Could you check a few things on this model? Use its own coordinates, in mm. A direction names the side the tool comes from. Round coordinates to 2 decimals unless told otherwise and drop trailing zeros. Write each loop counter-clockwise with the first axis right and the second up, starting at its lowest first coordinate (ties: lowest second). Pieces come first, ordered by that corner, then holes. Notation, with made-up numbers: (81.5, 5.5) -> (130.5, 5.5) arc R17 ccw to (130.5, 37.5) -> close; hole circle Ø3 at (-19, -26.5). An arc over 180 degrees is marked (long way). Answer as CSV lines item,"result". Start each with the question number.
Q1. If we mould it in two halves opening along X, with no side actions, what happens to faces 1 (the flat face through (-125.412, 2, 0)), 2 (the flat face through (-2, -125.412, 0)), 3 (the flat face through (-55, 118, 7.937)), 4 (the flat face through (122.238, -2, 2))? For each: pulls with the +X half, pulls with the -X half, needs draft (parallel to the pull), parting line crosses it, or undercut.
Q2. Imagine slicing it at A-A on x = -64.5. Please give me the cut outline in (y, z) (1 decimal).
Q3. If I drill on line 1 (X direction, y = 39.5, z = 7); line 2 (X direction, y = 22.5, z = 8.25) (3 decimals), over which ranges is the centre line in solid material (lowest first)? Write a range as [from, to].
Q4. Will these pins go through, and if not, where does the flat tip stop? pin 1 Ø5 at (y, z) = (-30, 1.5) entering from -X; pin 2 Ø6 at (y, z) = (-32, 1) entering from +X; pin 3 Ø1 at (x, z) = (41.5, -7) entering from +Y.
Q5. For faces 5 (the flat face through (125, -10, 11.112)), 6 (the flat face through (125.412, -2, 0)), 7 (the flat face through (-122.238, 2, 2)), 8 (the flat face through (2, 125.412, 0)), 9 (the flat face through (120, 10, -7.938)), which set-ups out of +Z, -Z, +X, -X, +Y, -Y let a thin tool reach every point of the face, with its end or its side?
Q6. Imagine slicing it at C-C on z = 0. Please give me the cut outline in (x, y), and give its area (3 significant figures).
from build123d import *


with BuildPart() as part:
    # Sweep1: sweep along a path in Sketch2
    with BuildLine(Plane.XY) as sweep1_path:
        Line((125.4125, -125.4125), (-125.4125, -125.4125))
        Line((-125.4125, -125.4125), (-125.4125, 125.4125))
        Line((-125.4125, 125.4125), (125.4125, 125.4125))
        Line((125.4125, 125.4125), (125.4125, -125.4125))
    # Sketch1 → Sweep1 (sweep)
    with BuildSketch(Plane(origin=(0, 0, 0), x_dir=(1, 0, 0), z_dir=(0, 1, 0))):
        Polygon((-125.4125, 7.9375), (-125.4125, -7.9375), (-130.175, -7.9375), (-130.175, -11.1125), (-117.475, -11.1125), (-117.475, -7.9375), (-122.2375, -7.9375), (-122.2375, 4.7625), (-117.475, 4.7625), (-117.475, 7.9375), align=None)
    sweep(path=sweep1_path.line, transition=Transition.RIGHT)


solid = part.part
Checks:
1,face 1,"pulls with the -X half"
1,face 2,"needs draft"
1,face 3,"undercut"
1,face 4,"undercut"
2,outline,"(-130.2, 7.9) -> (-125.4, 7.9) -> (-125.4, -7.9) -> (-117.5, -7.9) -> (-117.5, -4.8) -> (-122.2, -4.8) -> (-122.2, 7.9) -> (-117.5, 7.9) -> (-117.5, 11.1) -> (-130.2, 11.1) -> close; (117.5, -7.9) -> (125.4, -7.9) -> (125.4, 7.9) -> (130.2, 7.9) -> (130.2, 11.1) -> (117.5, 11.1) -> (117.5, 7.9) -> (122.2, 7.9) -> (122.2, -4.8) -> (117.5, -4.8) -> close"
3,line 1,"[-125.41, -122.24], [122.24, 125.41]"
3,line 2,"[-130.175, -117.475], [117.475, 130.175]"
4,pin 1,"x = -125.41"
4,pin 2,"x = 125.41"
4,pin 3,"y = 125.41"
5,face 5,"+Z, +X, -X, +Y, -Y"
5,face 6,"-Z, +X, +Y, -Y"
5,face 7,"none"
5,face 8,"-Z, +X, -X, +Y"
5,face 9,"-Z, +X, -X, +Y, -Y"
6,outline,"(-125.41, -125.41) -> (125.41, -125.41) -> (125.41, 125.41) -> (-125.41, 125.41) -> close; hole (-122.24, -122.24) -> (122.24, -122.24) -> (122.24, 122.24) -> (-122.24, 122.24) -> close"
6,area,"3,150 mm^2"
